Work out the finished part from the listing and answer in its coordinate system (mm). Round coordinates to 2 decimals unless told otherwise and drop trailing zeros. Order: outer loops, then holes, each group sorted by start corner. A loop starts at its lowest first (then second) coordinate and runs counter-clockwise, first axis right, second up. Notation, with made-up numbers: (32, 72.5) - (76, 72.5) arc R28 cw to (76, 110.5) - close; hole circle Ø7 at (-37, 0.25). An arc over 180 degrees is marked (long way). Answer in a Markdown table with one row per item.
from build123d import *

# Parameters (mm, degrees)
BOSS_EXTRUDE1_DEPTH = 34
SKETCH2_W           = 34
SKETCH2_H           = 15
BOSS_EXTRUDE2_DEPTH = 30
SKETCH3_R           = 10.25
CUT_EXTRUDE1_DEPTH  = 30
SKETCH4_W           = 20.5
SKETCH4_H           = 15
CUT_EXTRUDE2_DEPTH  = 34


with BuildPart() as part:
    # Sketch1 → Boss-Extrude1 (new body)
    # profile 1 of 3: a face of its own
    with BuildSketch(Plane.XY):
        with BuildLine():
            Line((-15, 0), (-15, -68))
            ThreePointArc((-15, -68), (0, -83), (15, -68))
            Line((15, -68), (15, 0))
            ThreePointArc((15, 0), (0, 15), (-15, 0))
        make_face()
        with BuildLine():
            ThreePointArc((-10.25, -68), (0, -78.25), (10.25, -68))
            Line((10.25, -68), (10.25, 0))
            ThreePointArc((10.25, 0), (0, 10.25), (-10.25, 0))
            Line((-10.25, 0), (-10.25, -68))
        make_face(mode=Mode.SUBTRACT)
    # profile 2 of 3: a face of its own
    with BuildSketch(Plane.XY):
        with BuildLine():
            Line((10.25, -68), (10.25, 0))
            ThreePointArc((10.25, 0), (0, -10.25), (-10.25, 0))
            Line((-10.25, 0), (-10.25, -68))
            ThreePointArc((-10.25, -68), (0, -57.75), (10.25, -68))
        make_face()
    # profile 3 of 3: a face of its own
    with BuildSketch(Plane.XY):
        with BuildLine():
            ThreePointArc((-10.25, -68), (0, -78.25), (10.25, -68))
            ThreePointArc((10.25, -68), (0, -57.75), (-10.25, -68))
        make_face()
    extrude(amount=BOSS_EXTRUDE1_DEPTH)

    # Sketch2 → Boss-Extrude2 (add)
    with BuildSketch(Plane.ZY.offset(15)):
        with Locations((17, -75.5)):
            Rectangle(SKETCH2_W, SKETCH2_H)
    extrude(amount=-BOSS_EXTRUDE2_DEPTH)

    # Sketch3 → Cut-Extrude1 (cut)
    with BuildSketch(Plane.ZY.offset(15)):
        with Locations(Location((17, -68, 0), (0, 0, 270))):
            Circle(SKETCH3_R)
    extrude(amount=-CUT_EXTRUDE1_DEPTH, mode=Mode.SUBTRACT)

    # Sketch4 → Cut-Extrude2 (cut)
    with BuildSketch(Plane.ZY.offset(15)):
        with Locations((17, -75.5)):
            Rectangle(SKETCH4_W, SKETCH4_H)
    extrude(amount=-CUT_EXTRUDE2_DEPTH, mode=Mode.SUBTRACT)


solid = part.part
1) Find the intervals of material crossed by probe 1 along Z at (x, y) = (8.5, -75); probe 2 along Y at (x, z) = (0, 23.5); probe 3 along Y at (x, z) = (-3.25, 24), in increasing order. Write a range as from..to.
Filled in:
| item | result |
|---|---|
| probe 1 | z = 0..6.75, 27.25..34 |
| probe 2 | y = -60.07..-10.25, 10.25..15 |
| probe 3 | y = -60.51..-9.72, 9.72..14.64 |
2) Find section D-D, the plane x = -11.5. Give the vertices of the cut face in (y, z), then the cut area to 3 significant figures.
Filled in:
| item | result |
|---|---|
| outline | (-83, 0) - (9.63, 0) - (9.63, 34) - (-83, 34) - (-83, 27.25) - (-68, 27.25) arc R10.25 cw to (-68, 6.75) - (-83, 6.75) - close |
| area | 2,680 mm^2 |
3) Find section B-B, the plane x = 7. Give the vertices of the cut face in (y, z).
Filled in:
| item | result |
|---|---|
| outline | (-83, 0) - (-7.49, 0) - (-7.49, 34) - (-83, 34) - (-83, 27.25) - (-68, 27.25) arc R10.25 cw to (-68, 6.75) - (-83, 6.75) - close; (7.49, 0) - (13.27, 0) - (13.27, 34) - (7.49, 34) - close |
4) Each of these flat-tipped pins is pushed along its axis until it touches: pin 1 (4 mm diameter, centred on x = 11.5, z = 9.5, fed in from +Y); pin 2 (1.5 mm diameter, centred on x = -6, y = -68.5, fed in from -Z). Where does it stop, or does it pass through?
Filled in:
| item | result |
|---|---|
| pin 1 | stops at y = 11.61 |
| pin 2 | stops at z = 0 |
5) Find section A-A, the plane y = -73. Give the vertices of the cut face in (x, z), then the cut area to 3 significant figures.
Filled in:
| item | result |
|---|---|
| outline | (-15, 0) - (15, 0) - (15, 6.75) - (-15, 6.75) - close; (-15, 27.25) - (15, 27.25) - (15, 34) - (-15, 34) - close |
| area | 405 mm^2 |
6) Find section C-C, the plane z = 17. Give the vertices of the cut face in (x, y), then the cut area to 3 significant figures.
Filled in:
| item | result |
|---|---|
| outline | (-15, -57.75) - (15, -57.75) - (15, 0) arc R15 ccw to (-15, 0) - close; hole circle Ø20.5 at (0, 0) |
| area | 1,760 mm^2 |
7) The mould has two halves that part along Z. Classify faces 1 (the face through (-15, -32, 17)), 2 (the face through (0, -46, 34)), 3 (the face through (0, -76, 6.75)), 4 (the face through (0, -76, 27.25)): released by +Z, released by -Z, zero draft, split by the parting line, or undercut.
Filled in:
| item | result |
|---|---|
| face 1 | zero draft |
| face 2 | released by +Z |
| face 3 | undercut |
| face 4 | undercut |
